Read the model definition and answer for the solid it produces. Units are mm, in the model's axes. A direction names the side the tool comes from. Coordinates: 2 decimals unless noted, no trailing zeros. Write each loop counter-clockwise with the first axis right and the second up, starting at its lowest first coordinate (ties: lowest second). Pieces come first, ordered by that corner, then holes.
(1) The part is cut by section C-C, the plane z = 35. Determine the outline of the cut face in (x, y), and give its area (3 significant figures).
(2) Determine the mould class of faces 3 (the flat face through (0, -9, 56)), 4 (the flat face through (95.25, -10, 89)), 5 (the flat face through (135, -9, 0)), 6 (the flat face through (273.05, -9, 56)) for opening direction X: pulls with the +X half, pulls with the -X half, needs draft (parallel to the pull), parting line crosses it, or undercut.
(3) The part is cut by section B-B, the plane x = 226. Determine the outline of the cut face in (y, z).
(4) Straight lines are drawn through the part: line 1 along X through (y, z) = (-17, 49); line 2 along X through (y, z) = (-13.25, 106); line 3 along X through (y, z) = (-1, 20). For each, find the intervals that lie inside material, in ascending order.
(5) The part is cut by section A-A, the plane y = -3.5. Determine the outline of the cut face in (x, z) (3 decimals).
(6) Given pin 1 (9.5 mm diameter, centred on x = 131, y = -7, fed in from +Z), flat-ended and moving along its own axis, determine where the tip first touches the part or whether it passes through.
(7) Which of the six approach directions +Z, -Z, +X, -X, +Y, -Y give full straight-line access (tool end or side, diameter ignored) to faces 1 (the flat face through (225, -9, 114.3)), 2 (the cylindrical face through (98.509, -9.658, 54.237))?
(8) The part is cut by section D-D, the plane x = 76. Determine the outline of the cut face in (y, z), and give its area (3 significant figures).
```python
from build123d import *

# Parameters (mm, degrees)
F0_W     = 273.05
F0_H     = 114.3
F1_DEPTH = 19.05
F2_R     = 38.1
F3_DEPTH = 25.4
F5_DEPTH = 25.4


with BuildPart() as f1:
    # F0 (on Front) → F1 (new body)
    with BuildSketch(Plane.XZ):
        with Locations((136.525, 57.15)):
            Rectangle(F0_W, F0_H)
    extrude(amount=F1_DEPTH)

    # F2 (on face) → F3 (cut)
    with BuildSketch(Plane.XZ.offset(19.05)):
        with Locations((225.425, 50.8)):
            Circle(F2_R)
        with Locations((47.625, 50.8)):
            Circle(F2_R)
    extrude(amount=-F3_DEPTH, mode=Mode.SUBTRACT)

    # F4 (on face) → F5 (cut)
    with BuildSketch(Plane.XZ.offset(19.05)):
        with BuildLine():
            Line((177.8, 114.3), (95.25, 114.3))
            Line((95.25, 114.3), (95.25, 62.23))
            ThreePointArc((95.25, 62.23), (98.597769, 54.147769), (106.68, 50.8))
            Line((106.68, 50.8), (166.37, 50.8))
            ThreePointArc((166.37, 50.8), (174.452231, 54.147769), (177.8, 62.23))
            Line((177.8, 62.23), (177.8, 114.3))
        make_face()
    extrude(amount=-F5_DEPTH, mode=Mode.SUBTRACT)


solid = f1.part
```
Computed:
1. outline: (0, -19.05) - (12.96, -19.05) - (12.96, 0) - (0, 0) - close; (82.29, -19.05) - (190.76, -19.05) - (190.76, 0) - (82.29, 0) - close; (260.09, -19.05) - (273.05, -19.05) - (273.05, 0) - (260.09, 0) - close
1. area: 2,560 mm2
2. face 3: pulls with the -X half
2. face 4: undercut
2. face 5: needs draft
2. face 6: pulls with the +X half
3. outline: (-19.05, 0) - (0, 0) - (0, 12.7) - (-19.05, 12.7) - close; (-19.05, 88.9) - (0, 88.9) - (0, 114.3) - (-19.05, 114.3) - close
4. line 1: x = 0 to 9.57, 85.68 to 187.37, 263.48 to 273.05
4. line 2: x = 0 to 95.25, 177.8 to 273.05
4. line 3: x = 0 to 25.2, 70.05 to 203, 247.85 to 273.05
5. outline: (0, 0) - (273.05, 0) - (273.05, 114.3) - (177.8, 114.3) - (177.8, 62.23) arc R11.43 cw to (166.37, 50.8) - (106.68, 50.8) arc R11.43 cw to (95.25, 62.23) - (95.25, 114.3) - (0, 114.3) - close; hole circle Ø76.2 at (47.625, 50.8); hole circle Ø76.2 at (225.425, 50.8)
6. pin 1: stops at z = 50.8
7. face 1: +Z, +X, -X, +Y, -Y
7. face 2: +Z, +Y, -Y
8. outline: (-19.05, 0) - (0, 0) - (0, 25.37) - (-19.05, 25.37) - close; (-19.05, 76.23) - (0, 76.23) - (0, 114.3) - (-19.05, 114.3) - close
8. area: 1,210 mm2
